Part print with two shaded views. Sizes in mm from the minimum x, y, z corner. A direction names the side the tool comes from. Round coordinates to 2 decimals unless told otherwise and drop trailing zeros. Loops run counter-clockwise (first coordinate to the right, second up) from the corner with the lowest first, then second, coordinate; pieces in that order, holes last. Notation, with made-up numbers: (51, 57) - (80, 57) arc R24 ccw to (80, 73) - close; hole circle Ø5 at (82.5, -19.5). An arc over 180 degrees is marked (long way). Write each question's results on one line, items separated by ' | '. Start each with the question number.
(1) Cut at D-D, the plane x = 195. List the corners of the cut face in (y, z).
(2) Tool access for the marked faces 1, 2 and 3: list every direction of +Z, -Z, +X, -X, +Y, -Y with a clear straight run to the whole face (end or side of a thin tool).
(3) Cut at A-A, the plane y = 56. List the corners of the cut face in (x, z), then the cut area to 3 significant figures.
(4) Flat gauge pins, fed straight in: P1, Ø6, axis at x = 109.5, y = 40, coming from the -Z side; P2, Ø2.5, axis at y = 40, z = 13.5, coming from the +X side; P3, Ø10, axis at y = 28, z = 15.5, coming from the -X side. Where does each tip first touch, or does it go through?
(5) Cut at C-C, the plane z = 12. List the corners of the cut face in (x, y).
(6) Cut at B-B, the plane x = 131. List the corners of the cut face in (y, z).
(7) Drill centre lines: L1, parallel to Y at x = 235, z = 24; L2, parallel to Z at x = 132.5, y = 40; L3, parallel to X at y = 36.5, z = 17. Where is each one in solid material? Low to high.
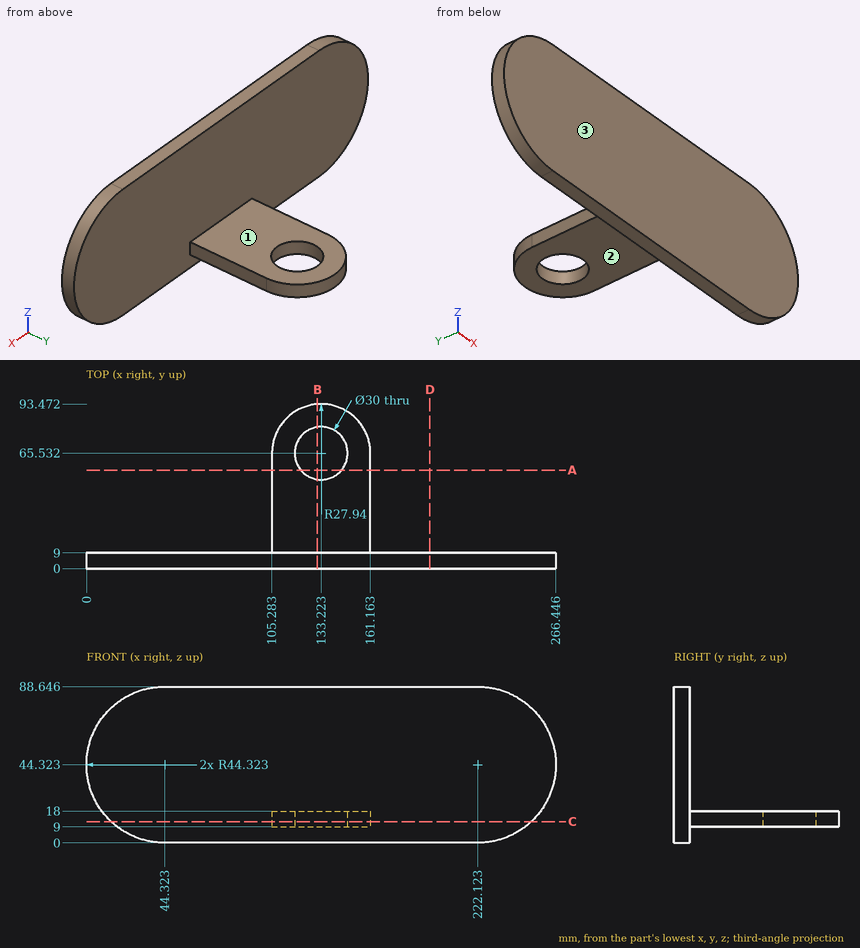
A:
1) outline: (0, 0) - (9, 0) - (9, 88.65) - (0, 88.65) - close
2) face 1: +Z, +X, -X, +Y | face 2: -Z, +X, -X, +Y | face 3: +Z, -Z, +X, -X, -Y
3) outline: (105.28, 9) - (121.64, 9) - (121.64, 18) - (105.28, 18) - close; (144.8, 9) - (161.16, 9) - (161.16, 18) - (144.8, 18) - close | area: 294 mm2
4) P1: z = 9 | P2: x = 161.16 | P3: x = 105.28
5) outline: (14, 0) - (252.45, 0) - (252.45, 9) - (161.16, 9) - (161.16, 65.53) arc R27.94 ccw to (105.28, 65.53) - (105.28, 9) - (14, 9) - close; hole circle Ø30 at (133.22, 65.53)
6) outline: (0, 0) - (9, 0) - (9, 9) - (50.7, 9) - (50.7, 18) - (9, 18) - (9, 88.65) - (0, 88.65) - close; (80.37, 9) - (93.38, 9) - (93.38, 18) - (80.37, 18) - close
7) L1: 0 to 9 | L2: 9 to 18 | L3: 105.28 to 161.16
